Could you check a few things on this model? Use its own coordinates, in mm. Give positions to 0.01 mm unless a question says otherwise; leave off trailing zeros. Write each loop counter-clockwise with the first axis right and the second up, starting at its lowest first coordinate (ties: lowest second). Pieces come first, ordered by that corner, then holes. Notation, with made-up numbers: M 58,-39.5 L 89,-39.5 A25 cw 89,-17.5 Z; hole C 29.5,-5.75 d5. An arc over 180 degrees is marked long. One line per item, written item: value.
```python
from build123d import *

# Parameters (mm, degrees)
SKETCH1_R           = 112
SKETCH1_W           = 3.1
SKETCH1_H           = 41
SKETCH1_W_2         = 4
SKETCH1_H_2         = 12
SKETCH1_H_3         = 10
BOSS_EXTRUDE1_DEPTH = 1.5


with BuildPart() as part:
    # Sketch1 → Boss-Extrude1 (new body, symmetric)
    with BuildSketch(Plane.XY):
        Circle(SKETCH1_R)
        with Locations((-60, 54.57272334)):
            Rectangle(SKETCH1_W, SKETCH1_H, mode=Mode.SUBTRACT)
        with Locations((-60, -54.57272334)):
            Rectangle(SKETCH1_W, SKETCH1_H, mode=Mode.SUBTRACT)
        with Locations((60, 54.57272334)):
            Rectangle(SKETCH1_W, SKETCH1_H, mode=Mode.SUBTRACT)
        with Locations((60, -54.57272334)):
            Rectangle(SKETCH1_W, SKETCH1_H, mode=Mode.SUBTRACT)
        with Locations((0, 7)):
            Rectangle(SKETCH1_W_2, SKETCH1_H_2, mode=Mode.SUBTRACT)
        with Locations((0, -7)):
            Rectangle(SKETCH1_W_2, SKETCH1_H_2, mode=Mode.SUBTRACT)
        with Locations((-10, 7)):
            Rectangle(SKETCH1_W_2, SKETCH1_H_3, mode=Mode.SUBTRACT)
        with Locations((-10, -7)):
            Rectangle(SKETCH1_W_2, SKETCH1_H_3, mode=Mode.SUBTRACT)
    extrude(amount=BOSS_EXTRUDE1_DEPTH, both=True)


solid = part.part
```
1) Please list where these lines run through material, in increasing order: L1, parallel to Y at x = 1.5, z = -1.3; L2, parallel to X at y = -46, z = -0.05; L3, parallel to X at y = 69.5, z = 0.3. Write a range as from..to.
Outcome:
L1: y = -111.99..-13, -1..1, 13..111.99
L2: x = -102.12..-61.55, -58.45..58.45, 61.55..102.12
L3: x = -87.83..-61.55, -58.45..58.45, 61.55..87.83
2) If we section it at B-B, the plane y = -41: Write out the boundary of the cut face in (x, z), then the cut area to 3 significant figures.
Outcome:
outline: M -104.23,-1.5 L -61.55,-1.5 L -61.55,1.5 L -104.23,1.5 Z; M -58.45,-1.5 L 58.45,-1.5 L 58.45,1.5 L -58.45,1.5 Z; M 61.55,-1.5 L 104.23,-1.5 L 104.23,1.5 L 61.55,1.5 Z
area: 607 mm^2
3) I'm going to push flat-ended pins straight in: pin 1 (1.5 mm diameter, centred on x = 59.5, z = 0.5, fed in from +Y); pin 2 (1.5 mm diameter, centred on y = -8.5, z = -0.5, fed in from +X); pin 3 (1.5 mm diameter, centred on y = 58.5, z = 0, fed in from +X). Where does each tip first touch, or does it pass through?
Outcome:
pin 1: stops at y = 95.35
pin 2: stops at x = 111.73
pin 3: stops at x = 95.96
4) If we section it at C-C, the plane x = 71: Write out the boundary of the cut face in (y, z).
Outcome:
outline: M -86.62,-1.5 L 86.62,-1.5 L 86.62,1.5 L -86.62,1.5 Z
5) If we section it at A-A, the plane z = -0.05: Give the number of separate pieces and of enclosed holes in the cut face, then the cut area to 3 significant figures.
Outcome:
separate pieces: 1
enclosed holes: 8
area: 38,700 mm^2
